Part model, mm, in its own coordinate system. A direction names the side the tool comes from. Give positions to 0.01 mm unless a question says otherwise; leave off trailing zeros. Loops run counter-clockwise (first coordinate to the right, second up) from the corner with the lowest first, then second, coordinate; pieces in that order, holes last. Notation, with made-up numbers: M 89,16.25 L 115,16.25 A7 cw 115,22.25 Z; hole C -12,34.5 d6. An arc over 180 degrees is marked long. Answer in a Markdown table with one row per item.
from build123d import *

# Parameters (mm, degrees)
F1_DEPTH  = 7.5
F2_T      = -1.5
F4_DEPTH  = 7.5
F6_DEPTH  = 2.9
F7_R      = 3.25
F8_DEPTH  = 50.001
F9_R      = 3.25
F10_DEPTH = 50.001


with BuildPart() as f1:
    # F0 (on Top) → F1 (new body)
    with BuildSketch(Plane.XY):
        Polygon((25, -8.75), (25, 8.75), (8.75, 8.75), (8.75, 25), (-8.75, 25), (-8.75, 8.75), (-25, 8.75), (-25, -8.75), (-8.75, -8.75), (-8.75, -25), (8.75, -25), (8.75, -8.75), align=None)
    extrude(amount=F1_DEPTH)

    # F2
    f2_openings = [f1.faces().sort_by_distance(p)[0] for p in [
        (0, 0, 7.5),
    ]]
    offset(amount=F2_T, openings=f2_openings, kind=Kind.INTERSECTION)

    # F3 (on face) → F4 (join, through all)
    with BuildSketch(Plane.XY.offset(7.5)):
        Polygon((-8.75, 11.5784271247), (-11.5784271247, 8.75), (-8.75, 8.75), align=None)
        Polygon((8.75, 11.5784271247), (8.75, 8.75), (11.5784271247, 8.75), align=None)
        Polygon((-8.75, -11.5784271247), (-8.75, -8.75), (-11.5784271247, -8.75), align=None)
        Polygon((11.5784271247, -8.75), (8.75, -8.75), (8.75, -11.5784271247), align=None)
    extrude(amount=-F4_DEPTH)

    # F5 (on face) → F6 (join)
    with BuildSketch(Plane.XY.offset(7.5)):
        with BuildLine():
            ThreePointArc((-9.5985281374, 9.5985281374), (-9.3714317932, 8.4568377178), (-8.4035533906, 9.1035533906))
            ThreePointArc((-8.4035533906, 9.1035533906), (-8.8356749879, 9.7502690634), (-9.5985281374, 9.5985281374))
        make_face()
        with BuildLine():
            ThreePointArc((9.5985281374, 9.5985281374), (8.4568377178, 8.8356749879), (9.8035533906, 9.1035533906))
            ThreePointArc((9.8035533906, 9.1035533906), (9.7502690634, 9.3714317932), (9.5985281374, 9.5985281374))
        make_face()
        with BuildLine():
            ThreePointArc((9.5985281374, -9.5985281374), (9.7502690634, -9.3714317932), (9.8035533906, -9.1035533906))
            ThreePointArc((9.8035533906, -9.1035533906), (8.4568377178, -8.8356749879), (9.5985281374, -9.5985281374))
        make_face()
        with BuildLine():
            ThreePointArc((-9.5985281374, -9.5985281374), (-8.8356749879, -9.7502690634), (-8.4035533906, -9.1035533906))
            ThreePointArc((-8.4035533906, -9.1035533906), (-9.3714317932, -8.4568377178), (-9.5985281374, -9.5985281374))
        make_face()
    extrude(amount=F6_DEPTH)

    # F7 (on face) → F8 (cut, through all)
    with BuildSketch(Plane.XZ.offset(25)):
        with Locations((0, 7.5)):
            Circle(F7_R)
    extrude(amount=-F8_DEPTH, mode=Mode.SUBTRACT)

    # F9 (on face) → F10 (cut, through all)
    with BuildSketch(Plane(origin=(-25, 0, 0), x_dir=(0, -1, 0), z_dir=(-1, 0, 0))):
        with Locations((0, 7.5)):
            Circle(F9_R)
    extrude(amount=-F10_DEPTH, mode=Mode.SUBTRACT)


solid = f1.part
(1) Saw through at A-A (z = 9.5). Write the cut outline in (x, y).
Recorded:
| item | result |
|---|---|
| outline | C -9.1,-9.1 d1.4; C -9.1,9.1 d1.4; C 9.1,-9.1 d1.4; C 9.1,9.1 d1.4 |
(2) Saw through at B-B (x = 0). Write the cut outline in (y, z), plus the area to 4 significant figures.
Recorded:
| item | result |
|---|---|
| outline | M -25,0 L 25,0 L 25,4.25 L 23.5,4.25 L 23.5,1.5 L -23.5,1.5 L -23.5,4.25 L -25,4.25 Z |
| area | 83.25 mm^2 |
(3) Saw through at C-C (y = 17). Write the cut outline in (x, z), plus the area to 4 significant figures.
Recorded:
| item | result |
|---|---|
| outline | M -8.75,0 L 8.75,0 L 8.75,7.5 L 7.25,7.5 L 7.25,1.5 L -7.25,1.5 L -7.25,7.5 L -8.75,7.5 Z |
| area | 44.25 mm^2 |
(4) Drill centre lines: line 1 along X through (y, z) = (-13.5, 4.25); line 2 along X through (y, z) = (7.5, 3). Where is each one in solid material? Low to high.
Recorded:
| item | result |
|---|---|
| line 1 | x = -8.75 to -7.25, 7.25 to 8.75 |
| line 2 | x = -25 to -7.25, 7.25 to 25 |
(5) Pull direction Y, two halves, no side cores. Call faces 4 (the face through (8.75, 18, 4)), 5 (the face through (18, -8.75, 4)), 6 (the face through (15, 7.25, 4)): +Y half, -Y half, draft (parallel to the pull), parting line (faces both ways), or undercut.
Recorded:
| item | result |
|---|---|
| face 4 | draft |
| face 5 | -Y half |
| face 6 | undercut |
(6) Pin check, flat tips, straight feed: pin 1 Ø6 at (x, z) = (-17.5, 3) entering from +Y; pin 2 Ø24 at (x, y) = (-10, -16.5) entering from +Z; pin 3 Ø4 at (x, z) = (-16, 2) entering from -Y; pin 4 Ø2 at (y, z) = (-19, 2) entering from -X. Stop position of each tip, or through.
Recorded:
| item | result |
|---|---|
| pin 1 | stops at y = 8.75 |
| pin 2 | stops at z = 10.4 |
| pin 3 | stops at y = -8.75 |
| pin 4 | stops at x = -8.75 |
(7) Saw through at D-D (z = 6.5). Give the number of separate pieces and of enclosed holes in the cut face, plus the area to 3 significant figures.
Recorded:
| item | result |
|---|---|
| separate pieces | 4 |
| enclosed holes | 0 |
| area | 270 mm^2 |
(8) Which spindle directions (+Z, -Z, +X, -X, +Y, -Y) get a long thin tool onto all of the face, cutting with end or side? Do faces 1 (the face through (-8.75, -18, 4)), 2 (the face through (-0.07, 24.24, 4.25)), 3 (the face through (-15, -7.25, 4)). Say none if no direction does.
Recorded:
| item | result |
|---|---|
| face 1 | +Z, -Z, -X, -Y |
| face 2 | +Z, +Y, -Y |
| face 3 | +Z |
